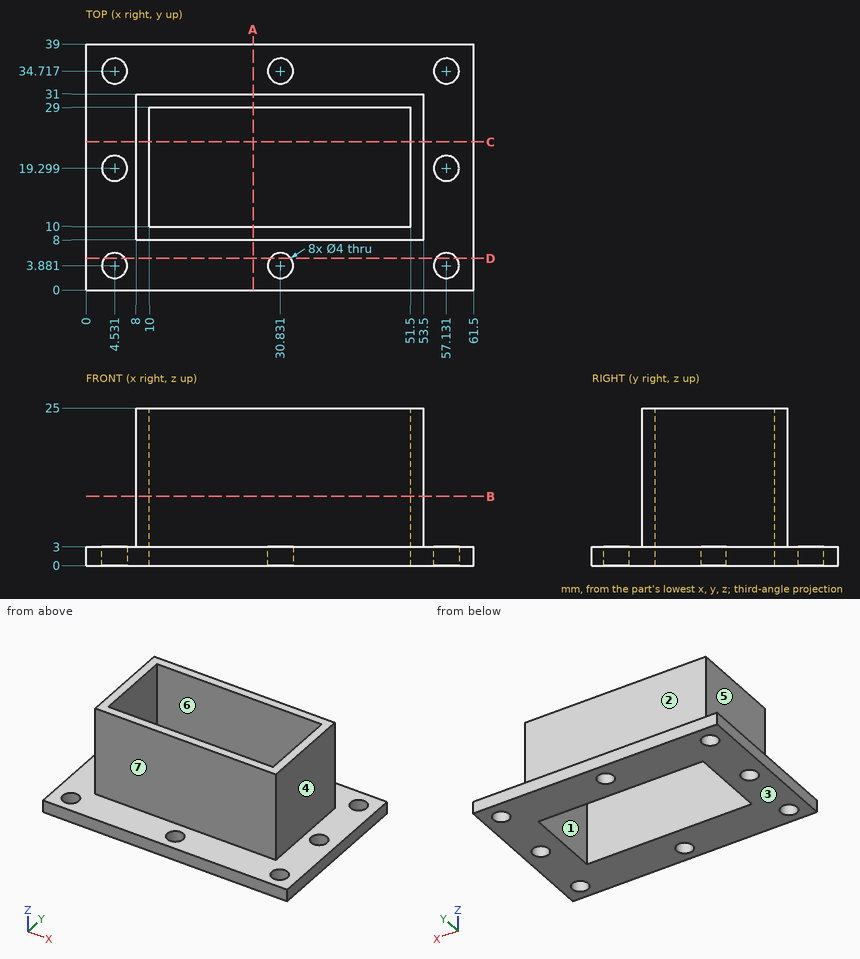
The drawing under review shows one solid part. Ordinate dimensions are in mm from its lowest x, y, z. A direction names the side the tool comes from. Round coordinates to 2 decimals unless told otherwise and drop trailing zeros. Write each loop counter-clockwise with the first axis right and the second up, starting at its lowest first coordinate (ties: lowest second). Pieces come first, ordered by that corner, then holes. Notation, with made-up numbers: (31.25, 13) - (71.25, 13) arc R30 ccw to (71.25, 37) - close; hole circle Ø11 at (-29, 2.5). An arc over 180 degrees is marked (long way). Use one line per item in the form item = value.
Q1. Consider section D-D (y = 5). State the section outline as (x, z) points, and give its area (3 significant figures).
Answer key:
outline = (0, 0) - (2.87, 0) - (2.87, 3) - (0, 3) - close; (6.19, 0) - (29.17, 0) - (29.17, 3) - (6.19, 3) - close; (32.49, 0) - (55.47, 0) - (55.47, 3) - (32.49, 3) - close; (58.79, 0) - (61.5, 0) - (61.5, 3) - (58.79, 3) - close
area = 155 mm2
Q2. For line 1 (Y direction, x = 49, z = 12.25); line 2 (X direction, y = 23, z = 16.5); line 3 (Z direction, x = 55, y = 8), list the stretches that pass through material, from the lowest coordinate up. Write a range as [from, to].
Answer key:
line_1 = [8, 10], [29, 31]
line_2 = [8, 10], [51.5, 53.5]
line_3 = [0, 3]
Q3. Consider section C-C (y = 23.5). State the section outline as (x, z) points.
Answer key:
outline = (0, 0) - (10, 0) - (10, 25) - (8, 25) - (8, 3) - (0, 3) - close; (51.5, 0) - (61.5, 0) - (61.5, 3) - (53.5, 3) - (53.5, 25) - (51.5, 25) - close
Q4. Consider section B-B (z = 11). State the section outline as (x, y) points, and give its area (3 significant figures).
Answer key:
outline = (8, 8) - (53.5, 8) - (53.5, 31) - (8, 31) - close; hole (10, 10) - (51.5, 10) - (51.5, 29) - (10, 29) - close
area = 258 mm2
Q5. Draft analysis for pull direction X (two halves, no side actions). For the marked faces 5, 6 and 7, state which applies: +X half, -X half, draft (parallel to the pull), parting line (faces both ways), or undercut.
Answer key:
face_5 = -X half
face_6 = undercut
face_7 = draft
Q6. Consider section A-A (x = 26.5). State the section outline as (y, z) points.
Answer key:
outline = (0, 0) - (10, 0) - (10, 25) - (8, 25) - (8, 3) - (0, 3) - close; (29, 0) - (39, 0) - (39, 3) - (31, 3) - (31, 25) - (29, 25) - close
Q7. Tool access review of the marked faces 1, 2, 3 and 4: name each direction out of +Z, -Z, +X, -X, +Y, -Y from which nothing blocks a thin tool from reaching the whole face with its end or side.
Answer key:
face_1 = +Z, -Z
face_2 = +Z, +X, -X, +Y
face_3 = -Z, +X, -X, +Y, -Y
face_4 = +Z, +X, +Y, -Y
Q8. Insertion check: pin 1 Ø11 at (x, z) = (25.5, 13.5) entering from +Y; pin 2 Ø10 at (x, y) = (26, 28.5) entering from +Z; pin 3 Ø6.5 at (x, y) = (4.53, 3.88) entering from +Z; pin 4 Ø2 at (y, z) = (15, 7) entering from -X. Each pin has a flat end and moves straight along its axis. Give the tip position at first contact, or say it passes through.
Answer key:
pin_1 = 31
pin_2 = 25
pin_3 = 3
pin_4 = 8
